For this review, take the finished solid that the model builds, in its own axes (mm). A direction names the side the tool comes from. Coordinates: 2 decimals unless noted, no trailing zeros. Write each loop counter-clockwise with the first axis right and the second up, starting at its lowest first coordinate (ties: lowest second). Pieces come first, ordered by that corner, then holes.
```python
from build123d import *

# Parameters (mm, degrees)
SKETCH1_W           = 15
SKETCH1_H           = 15
BOSS_EXTRUDE1_DEPTH = 75
BOSS_EXTRUDE1_TAPER = 1.5
SKETCH2_R           = 1.5
CUT_EXTRUDE1_DEPTH  = 10
SKETCH3_R           = 2.75
CUT_EXTRUDE2_DEPTH  = 2
FILLET1_R           = 1.5
FILLET2_R           = 0.5


with BuildPart() as part:
    # Sketch1 → Boss-Extrude1 (new body)
    with BuildSketch(Plane.XY):
        Rectangle(SKETCH1_W, SKETCH1_H)
    extrude(amount=BOSS_EXTRUDE1_DEPTH, taper=BOSS_EXTRUDE1_TAPER)

    # Sketch2 → Cut-Extrude1 (cut)
    with BuildSketch(Plane(origin=(0, 0, 0), x_dir=(-1, 0, 0), z_dir=(0, 0, -1))):
        Circle(SKETCH2_R)
    extrude(amount=-CUT_EXTRUDE1_DEPTH, mode=Mode.SUBTRACT)

    # Sketch3 → Cut-Extrude2 (cut)
    with BuildSketch(Plane.XY.offset(75)):
        Circle(SKETCH3_R)
    extrude(amount=-CUT_EXTRUDE2_DEPTH, mode=Mode.SUBTRACT)

    # Fillet1
    fillet1_edges = [part.edges().sort_by_distance(p)[0] for p in [
        (-5.536055882, 0, 75),
        (0, -5.536055882, 75),
        (5.536055882, 0, 75),
        (6.518027941, -6.518027941, 37.5),
        (-6.518027941, -6.518027941, 37.5),
        (-6.518027479, 6.518027479, 37.500017641),
        (6.518027941, 6.518027941, 37.5),
        (0, 5.536055882, 75),
    ]]
    fillet(fillet1_edges, radius=FILLET1_R)

    # Fillet2
    fillet2_edges = [part.edges().sort_by_distance(p)[0] for p in [
        (1.5, 0, 0),
    ]]
    fillet(fillet2_edges, radius=FILLET2_R)


solid = part.part
```
Q1. Draft analysis for pull direction X (two halves, no side actions). For faces 4 (the cylindrical face through (1.5, 0.07, 5.18)), 5 (the cylindrical face through (6.07, -6.1, 37.29)), 6 (the cylindrical face through (-0.596, -2.685, 74.014)), 7 (the cylindrical face through (-0.057, 5.133, 74.563)), state which applies: +X half, -X half, draft (parallel to the pull), parting line (faces both ways), or undercut.
Ans:
face 4: undercut
face 5: +X half
face 6: undercut
face 7: draft
Q2. Clearance check with flat-ended pins moving along their axes: pin 1 Ø3 at (x, z) = (-5.5, 45.5) entering from +Y; pin 2 Ø4 at (x, y) = (0, 0) entering from +Z; pin 3 Ø6 at (x, z) = (2.5, 12.5) entering from +Y. State where each tip first meets the part, or that it passes through.
Ans:
pin 1: stops at y = 6.34
pin 2: stops at z = 73
pin 3: stops at y = 7.25
Q3. Tool access review of faces 1 (the flat face through (0, 3, 75)), 2 (the flat face through (0, 0, 73)), 3 (the flat face through (0, 0, 10)): name each direction out of +Z, -Z, +X, -X, +Y, -Y from which nothing blocks a thin tool from reaching the whole face with its end or side.
Ans:
face 1: +Z, +X, -X, +Y, -Y
face 2: +Z
face 3: -Z
Q4. Add section A-A (y = 0). State the section outline as (x, z) points, then the cut area to 3 significant figures.
Ans:
outline: (-7.5, 0) - (-2, 0) arc R0.5 ccw to (-1.5, 0.5) - (-1.5, 10) - (1.5, 10) - (1.5, 0.5) arc R0.5 ccw to (2, 0) - (7.5, 0) - (5.57, 73.54) arc R1.5 ccw to (4.07, 75) - (2.75, 75) - (2.75, 73) - (-2.75, 73) - (-2.75, 75) - (-4.07, 75) arc R1.5 ccw to (-5.57, 73.54) - close
area: 936 mm2
Q5. For probe 1 along Z at (x, y) = (0.75, 0.75); probe 2 along Z at (x, y) = (2.5, -0.75); probe 3 along Y at (x, z) = (0, 74.3), list the stretches that pass through material, from the lowest coordinate up.
Ans:
probe 1: z = 10 to 73
probe 2: z = 0 to 73
probe 3: y = -5.34 to -2.75, 2.75 to 5.34
